Geometry check sheet. Reference: the model listing, model coordinates, mm. A direction names the side the tool comes from. Round coordinates to 2 decimals unless told otherwise and drop trailing zeros. Loops run counter-clockwise (first coordinate to the right, second up) from the corner with the lowest first, then second, coordinate; pieces in that order, holes last. Notation, with made-up numbers: M -8,22 L 19,22 A18 cw 19,57 Z; hole C -2,-31.5 d7. An arc over 180 degrees is marked long. Write item = value, one per line.
from build123d import *

# Parameters (mm, degrees)
F0_W     = 140
F0_H     = 60
F1_DEPTH = 7.5
F2_R     = 3
F3_W     = 7.2
F3_H     = 7.2
F3_H_2   = 4.9
F4_DEPTH = 3.5
F3_H_3   = 11.5
F5_DEPTH = 10
F6_DEPTH = 25
F7_START = 4
F7_DEPTH = 6


with BuildPart() as f1:
    # F0 (on Top) → F1 (new body)
    with BuildSketch(Plane.XY):
        Rectangle(F0_W, F0_H)
    extrude(amount=F1_DEPTH)

    # F2
    f2_edges = [f1.edges().sort_by_distance(p)[0] for p in [
        (0, -30, 7.5),
        (70, 0, 7.5),
        (0, 30, 7.5),
        (-70, 0, 7.5),
        (0, 30, 0),
        (70, 30, 3.75),
        (70, 0, 0),
        (70, -30, 3.75),
        (-70, 30, 3.75),
        (-70, 0, 0),
        (0, -30, 0),
        (-70, -30, 3.75),
    ]]
    fillet(f2_edges, radius=F2_R)

    # F3 (on Top) → F4 (cut)
    with BuildSketch(Plane.XY):
        with Locations((0, -7)):
            Rectangle(F3_W, F3_H)
        with Locations((0, -24.55)):
            Rectangle(F3_W, F3_H_2)
    extrude(amount=F4_DEPTH, mode=Mode.SUBTRACT)

    # F3 (on Top) → F5 (cut)
    with BuildSketch(Plane.XY):
        with Locations((0, -16.35)):
            Rectangle(F3_W, F3_H_3)
    extrude(amount=F5_DEPTH, mode=Mode.SUBTRACT)

    # F3 (on Top) → F6 (cut)
    with BuildSketch(Plane.XY):
        with Locations((-11.8, -16.35)):
            Rectangle(F3_W, F3_H_3)
        with Locations((11.8, -16.3500007004)):
            Rectangle(F3_W, F3_H_3)
    extrude(amount=F6_DEPTH, mode=Mode.SUBTRACT)

    # F3 (on Top) → F7 (cut)
    with BuildSketch(Plane.XY.offset(F7_START)):
        with Locations((-11.8, -24.55)):
            Rectangle(F3_W, F3_H_2)
        with Locations((-11.8, -7)):
            Rectangle(F3_W, F3_H)
        with Locations((11.8, -7.0000007004)):
            Rectangle(F3_W, F3_H)
        with Locations((11.8, -24.5500007004)):
            Rectangle(F3_W, F3_H_2)
    extrude(amount=F7_DEPTH, mode=Mode.SUBTRACT)


solid = f1.part
(1) Sectioned sample at A-A on x = -12.5. Record the cut outline in (y, z).
Result set:
outline = M -30,3 A3 ccw -27,0 L -22.1,0 L -22.1,4 L -27,4 L -27,7.5 A3 ccw -30,4.5 Z; M -10.6,0 L 27,0 A3 ccw 30,3 L 30,4.5 A3 ccw 27,7.5 L -3.4,7.5 L -3.4,4 L -10.6,4 Z
(2) Sectioned sample at B-B on z = 6. Record the cut outline in (x, y).
Result set:
outline = M -69.6,-27 A2.6 ccw -67,-29.6 L 67,-29.6 A2.6 ccw 69.6,-27 L 69.6,27 A2.6 ccw 67,29.6 L -67,29.6 A2.6 ccw -69.6,27 Z; hole M -15.4,-27 L -8.2,-27 L -8.2,-3.4 L -15.4,-3.4 Z; hole M -3.6,-22.1 L 3.6,-22.1 L 3.6,-10.6 L -3.6,-10.6 Z; hole M 8.2,-27 L 15.4,-27 L 15.4,-3.4 L 8.2,-3.4 Z
(3) Release check for a two-part mould opening along Y. For faces 4 (the cylindrical face through (0.94, -29.14, 6.6)), 5 (the flat face through (15.4, -15, 5)), 6 (the flat face through (-1, 0, 7.5)) record: released by +Y, released by -Y, zero draft, split by the parting line, or undercut.
Result set:
face_4 = released by -Y
face_5 = undercut
face_6 = zero draft
(4) Tool access check on faces 1 (the flat face through (0, -10.6, 5)), 2 (the cylindrical face through (-69.14, 0.38, 6.6)), 3 (the flat face through (12, -7, 4)). Record the directions out of +Z, -Z, +X, -X, +Y, -Y that give a thin tool (end or side, any length) a straight path to the whole face; none if there is none.
Result set:
face_1 = +Z, -Z
face_2 = +Z, -X, +Y, -Y
face_3 = +Z
(5) Material ranges on line 1 along X through (y, z) = (-9.5, 4.5); line 2 along X through (y, z) = (-10.5, 3); line 3 along X through (y, z) = (-11.5, 1.25), recorded low to high. Write a range as from..to.
Result set:
line_1 = -70..-15.4, -8.2..8.2, 15.4..70
line_2 = -70..-3.6, 3.6..70
line_3 = -69.44..-15.4, -8.2..-3.6, 3.6..8.2, 15.4..69.44
(6) Depth check by flat-ended pin: pin 1 Ø2 at (x, y) = (-12, -8.5) entering from +Z; pin 2 Ø1.7 at (x, z) = (11.5, 5.5) entering from +Y; pin 3 Ø1.2 at (x, z) = (0, 6.5) entering from +Y; pin 4 Ø3 at (x, z) = (0, 1.5) entering from -Y. Enter the tip coordinate at first touch or a pass-through.
Result set:
pin_1 = 4
pin_2 = 30
pin_3 = 29.65
pin_4 = -30
(7) Sectioned sample at C-C on x = 23. Record the cut outline in (y, z), then the cut area to 3 significant figures.
Result set:
outline = M -30,3 A3 ccw -27,0 L 27,0 A3 ccw 30,3 L 30,4.5 A3 ccw 27,7.5 L -27,7.5 A3 ccw -30,4.5 Z
area = 442 mm2
